Design review of the part built by this model. Coordinates are the model's own, in mm. A direction names the side the tool comes from. Give positions to 0.01 mm unless a question says otherwise; leave off trailing zeros. Write each loop counter-clockwise with the first axis right and the second up, starting at its lowest first coordinate (ties: lowest second). Pieces come first, ordered by that corner, then holes. Notation, with made-up numbers: M 83,-10.5 L 124,-10.5 A21 cw 124,28.5 Z; hole C 53,32.5 d7. An arc over 180 degrees is marked long. Answer in a Markdown table with one row per item.
```python
from build123d import *

# Parameters (mm, degrees)
SKETCH1_W                  = 420
SKETCH1_H                  = 297
PLATE_DEPTH                = 6
TAPPED_HOLES_M4_DEPTH      = 258.270771756
TAPPED_HOLES_M4_DEPTH_BACK = 258.270771756
SKETCH2_R                  = 1.65
JAR_LOCATING_RINGS_START   = 6
SKETCH3_R                  = 48.5
SKETCH3_R_2                = 45.5
JAR_LOCATING_RINGS_DEPTH   = 2


with BuildPart() as part:
    # Sketch1 → Plate (new body)
    with BuildSketch(Plane(origin=(0, 0, 0), x_dir=(1, 0, 0), z_dir=(0, 1, 0))):
        Rectangle(SKETCH1_W, SKETCH1_H)
    extrude(amount=PLATE_DEPTH)

    # Sketch2 → Tapped_Holes_M4 (cut, two sides: drawn at the far end of the back side and taken through both)
    with BuildSketch(Plane(origin=(0, 0, 0), x_dir=(1, 0, 0), z_dir=(0, 1, 0)).offset(-TAPPED_HOLES_M4_DEPTH_BACK)):
        with Locations(Location((-97, -108, 0), (0, 0, 270))):
            Circle(SKETCH2_R)
        with Locations(Location((71, -108, 0), (0, 0, 270))):
            Circle(SKETCH2_R)
        with Locations(Location((-180, 117, 0), (0, 0, 270))):
            Circle(SKETCH2_R)
        with Locations(Location((-180, 93, 0), (0, 0, 270))):
            Circle(SKETCH2_R)
        with Locations(Location((-10, 117, 0), (0, 0, 270))):
            Circle(SKETCH2_R)
        with Locations(Location((-10, 93, 0), (0, 0, 270))):
            Circle(SKETCH2_R)
        with Locations(Location((109.5, -65.85, 0), (0, 0, 270))):
            Circle(SKETCH2_R)
        with Locations(Location((109.5, -124.15, 0), (0, 0, 270))):
            Circle(SKETCH2_R)
        with Locations(Location((140.5, -65.85, 0), (0, 0, 270))):
            Circle(SKETCH2_R)
        with Locations(Location((140.5, -124.15, 0), (0, 0, 270))):
            Circle(SKETCH2_R)
        with Locations(Location((158.3225, 18, 0), (0, 0, 270))):
            Circle(SKETCH2_R)
        with Locations(Location((201.6775, 18, 0), (0, 0, 270))):
            Circle(SKETCH2_R)
        with Locations(Location((76.5, -18.3225, 0), (0, 0, 270))):
            Circle(SKETCH2_R)
        with Locations(Location((76.5, -61.6775, 0), (0, 0, 270))):
            Circle(SKETCH2_R)
    extrude(amount=TAPPED_HOLES_M4_DEPTH + TAPPED_HOLES_M4_DEPTH_BACK, mode=Mode.SUBTRACT)

    # Sketch3 → Jar_Locating_Rings (add)
    # profile 1 of 3: a face of its own
    with BuildSketch(Plane(origin=(0, 0, 0), x_dir=(1, 0, 0), z_dir=(0, 1, 0)).offset(JAR_LOCATING_RINGS_START)):
        with Locations(Location((-160, -95, 0), (0, 0, 270))):
            Circle(SKETCH3_R)
        with Locations(Location((-160, -95, 0), (0, 0, 270))):
            Circle(SKETCH3_R_2, mode=Mode.SUBTRACT)
    # profile 2 of 3: a face of its own
    with BuildSketch(Plane(origin=(0, 0, 0), x_dir=(1, 0, 0), z_dir=(0, 1, 0)).offset(JAR_LOCATING_RINGS_START)):
        with Locations(Location((35, 35, 0), (0, 0, 90))):
            Circle(SKETCH3_R)
        with Locations(Location((35, 35, 0), (0, 0, 270))):
            Circle(SKETCH3_R_2, mode=Mode.SUBTRACT)
    # profile 3 of 3: a face of its own
    with BuildSketch(Plane(origin=(0, 0, 0), x_dir=(1, 0, 0), z_dir=(0, 1, 0)).offset(JAR_LOCATING_RINGS_START)):
        with Locations(Location((110, 100, 0), (0, 0, 90))):
            Circle(SKETCH3_R)
        with Locations(Location((110, 100, 0), (0, 0, 270))):
            Circle(SKETCH3_R_2, mode=Mode.SUBTRACT)
    extrude(amount=JAR_LOCATING_RINGS_DEPTH)


solid = part.part
```
1) To check wall thickness, follow probe 1 along Z at (x, y) = (109.5, 2); probe 2 along X at (y, z) = (1.25, -92.5); probe 3 along X at (y, z) = (3.85, 124.15). State the ranges of each line that lie inside material, in increasing order. Write a range as [from, to].
Geometry says:
| item | result |
|---|---|
| probe 1 | [-148.5, 64.2], [67.5, 122.5], [125.8, 148.5] |
| probe 2 | [-210, -181.57], [-178.43, -11.57], [-8.43, 210] |
| probe 3 | [-210, 107.85], [111.15, 138.85], [142.15, 210] |
2) For faces 1 (the face through (-145.4, 8, 51.7)), 2 (the face through (-161, 6, 94)), list the 3-axis set-ups (+Z, -Z, +X, -X, +Y, -Y) from which the entire face can be reached by the end or side of a thin tool; tool diameter is ignored.
Geometry says:
| item | result |
|---|---|
| face 1 | +Z, -Z, +X, -X, +Y |
| face 2 | +Y |
3) Insertion check: P1, Ø2, axis at x = 71, z = 108, coming from the -Y side; P2, Ø5, axis at x = 160, z = 30.5, coming from the +Y side. Each pin has a flat end and moves straight along its axis. Give the tip position at first contact, or say it passes through.
Geometry says:
| item | result |
|---|---|
| P1 | through |
| P2 | y = 6 |
4) Add section A-A (x = 35). Write out the cut boundary in (y, z).
Geometry says:
| item | result |
|---|---|
| outline | M 0,-148.5 L 6,-148.5 L 6,-83.5 L 8,-83.5 L 8,-80.5 L 6,-80.5 L 6,10.5 L 8,10.5 L 8,13.5 L 6,13.5 L 6,148.5 L 0,148.5 Z |
5) The part is to be moulded in two halves that separate along Z. For faces 3 (the face through (-129.249, 6.986, 61.465)), 4 (the face through (109, 6, -101)), 5 (the face through (-3, 0, -2)), 6 (the face through (-207.347, 6.986, 84.486)), say which applies: released by +Z, released by -Z, zero draft, split by the parting line, or undercut.
Geometry says:
| item | result |
|---|---|
| face 3 | undercut |
| face 4 | undercut |
| face 5 | zero draft |
| face 6 | split by the parting line |
6) Add section B-B (z = -35). Write out the cut boundary in (x, y).
Geometry says:
| item | result |
|---|---|
| outline | M -210,0 L 210,0 L 210,6 L 83.5,6 L 83.5,8 L 80.5,8 L 80.5,6 L -10.5,6 L -10.5,8 L -13.5,8 L -13.5,6 L -210,6 Z |
7) Add section C-C (x = -67). Write out the cut boundary in (y, z).
Geometry says:
| item | result |
|---|---|
| outline | M 0,-148.5 L 6,-148.5 L 6,148.5 L 0,148.5 Z |
